Build history of the part. All positions in model axes, mm. Face numbers are marked on the shaded views. A direction names the side the tool comes from. Give positions to 0.01 mm unless a question says otherwise; leave off trailing zeros. Order: outer loops, then holes, each group sorted by start corner. A loop starts at its lowest first (then second) coordinate and runs counter-clockwise, first axis right, second up. Notation, with made-up numbers: (66, 3.5) - (121, 3.5) arc R28 cw to (121, 21.5) - close; hole circle Ø7 at (-33, -23.75). An arc over 180 degrees is marked (long way). Use a Markdown table: item, result. Add a question column.
(1) Wall check: line 1 (Y direction, x = -0.4, z = 0.9); line 2 (Z direction, x = 0.1, y = -2); line 3 (Y direction, x = 0.1, z = 1.95). Give the ranges that are in metal, low to high.
(2) Mould opens along Z. For the marked faces 3, 4 and 5 say: +Z half, -Z half, draft (parallel to the pull), parting line (faces both ways), or undercut.
(3) Slice it at A-A (y = -6.25). Write the cut outline in (x, z), then the cut area to 3 significant figures.
(4) Which spindle directions (+Z, -Z, +X, -X, +Y, -Y) get a long thin tool onto all of the face, cutting with end or side? Do the marked faces 1 and 2. Say none if no direction does.
(5) Flat gauge pins, fed straight in: pin 1 (3 mm diameter, centred on x = 2, z = -2, fed in from +Y); pin 2 (3 mm diameter, centred on y = -13, z = -1.5, fed in from +X); pin 3 (1.2 mm diameter, centred on x = 0, z = 0.5, fed in from +Y); pin 4 (2 mm diameter, centred on x = -1, y = -7.5, fed in from +Z). Where does each tip first touch, or does it go through?
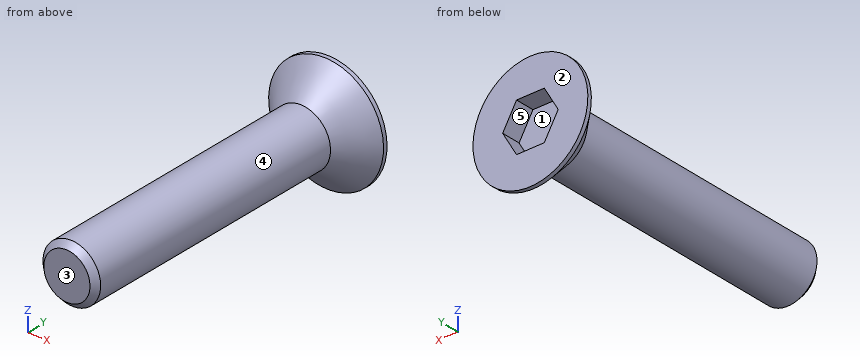
from build123d import *

# Parameters (mm, degrees)
CHAFL_N2_SIZE         = 0.3
CHAFL_N2_SIZE2        = 0.212132034
CHAFL_N3_SIZE         = 0.3
CORTAR_EXTRUIR2_DEPTH = 1


with BuildPart() as part:
    # Croquis1 → Revolución1 (revolve)
    with BuildSketch(Plane.XY, mode=Mode.PRIVATE) as revoluci_n1_sk:
        Polygon((0, 0), (3.2, 0), (1.5, -1.7), (1.5, -16), (0, -16), align=None)
    revolve(revoluci_n1_sk.sketch.rotate(Axis((0, 0, 0), (0, -1, 0)), 90), axis=Axis((0, 0, 0), (0, -1, 0)))

    # Chaflán2
    chafl_n2_edges = [part.edges().sort_by_distance(p)[0] for p in [
        (0, 0, -3.2),
    ]]
    chafl_n2_side = [part.faces().sort_by_distance(p)[0] for p in [
        (0, -0.85, -2.35),
    ]]
    chamfer(chafl_n2_edges, length=CHAFL_N2_SIZE, length2=CHAFL_N2_SIZE2, reference=chafl_n2_side[0])

    # Chaflán3
    chafl_n3_edges = [part.edges().sort_by_distance(p)[0] for p in [
        (0, -16, -1.5),
    ]]
    chamfer(chafl_n3_edges, length=CHAFL_N3_SIZE)

    # Croquis3 → Cortar-Extruir2 (cut)
    with BuildSketch(Plane(origin=(0, 0, 0), x_dir=(1, 0, 0), z_dir=(0, 1, 0))):
        Polygon((-0.721687836, 1.25), (-1.443375673, 0), (-0.721687836, -1.25), (0.721687836, -1.25), (1.443375673, 0), (0.721687836, 1.25), align=None)
    extrude(amount=-CORTAR_EXTRUIR2_DEPTH, mode=Mode.SUBTRACT)


solid = part.part
Solution:
| question | item | result |
|---|---|---|
| 1 | line 1 | -16 to -1 |
| 1 | line 2 | -1.5 to 1.5 |
| 1 | line 3 | -1.25 to 0 |
| 2 | face 3 | draft |
| 2 | face 4 | parting line |
| 2 | face 5 | undercut |
| 3 | outline | circle Ø3 at (0, 0) |
| 3 | area | 7.07 mm2 |
| 4 | face 1 | +Y |
| 4 | face 2 | +Z, -Z, +X, -X, +Y |
| 5 | pin 1 | y = 0 |
| 5 | pin 2 | x = 1.5 |
| 5 | pin 3 | y = -1 |
| 5 | pin 4 | z = 1.5 |
